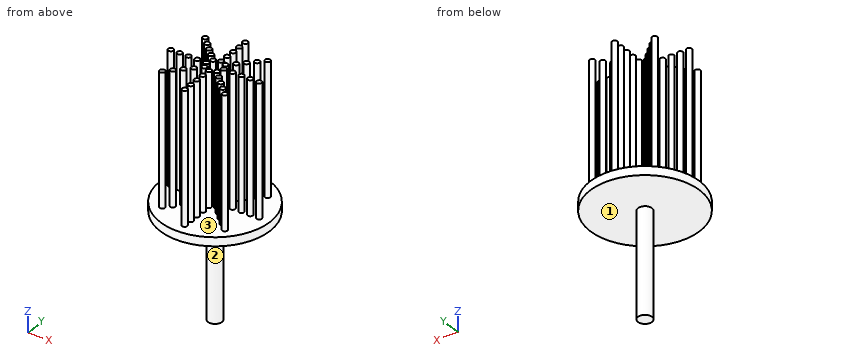
```python
from build123d import *

# Parameters (mm, degrees)
F0_R            = 62.5
F1_DEPTH        = 10
F2_R            = 3
F3_DEPTH        = 150
F3_COPIES_COUNT = 8
F4_R            = 8
F5_DEPTH        = 120


# Not quite as in the source:
# - a pattern or mirror of a feature is missing from the dataset's text; its kind, count and spacing are read off the source's solid


with BuildPart() as f1:
    # F0 (on Top) → F1 (new body)
    with BuildSketch(Plane.XY):
        Circle(F0_R)
    extrude(amount=F1_DEPTH)

    # F2 (on face) → F3 (join)
    with BuildSketch(Plane.XY.offset(10)):
        with Locations((10, 0)):
            Circle(F2_R)
        with Locations((20, 0)):
            Circle(F2_R)
        with Locations((30, 0)):
            Circle(F2_R)
        with Locations((40, 0)):
            Circle(F2_R)
        with Locations((50, 0)):
            Circle(F2_R)
    f3 = extrude(amount=F3_DEPTH)

    # F3_copies: F3 ×8 about axis
    f3_copies_axis = Axis((0, 0, 0), (0, 0, 1))
    for i in range(1, F3_COPIES_COUNT):
        add(f3.rotate(f3_copies_axis, i * 360 / F3_COPIES_COUNT))

    # F4 (on face) → F5 (join)
    with BuildSketch(Plane.XY):
        Circle(F4_R)
    extrude(amount=-F5_DEPTH)


solid = f1.part
```
Verification items for the finished model (mm, model axes). Face numbers are marked on the shaded views. Coordinates: 2 decimals unless noted, no trailing zeros. Order: outer loops, then holes, each group sorted by start corner. A loop starts at its lowest first (then second) coordinate and runs counter-clockwise, first axis right, second up. Notation, with made-up numbers: (87.5, 77.25) -> (126.5, 77.25) arc R21 cw to (126.5, 85.25) -> close; hole circle Ø3 at (-3, 19.25). An arc over 180 degrees is marked (long way). Answer as CSV lines item,"result". Start each with the question number.
1) Cross-section at C-C, the plane z = 104. Give the number of separate pieces and of enclosed holes in the cut face, then the cut area to 3 significant figures.
2) Release check for a two-part mould opening along Y. For the marked faces 1, 2 and 3 record: released by +Y, released by -Y, zero draft, split by the parting line, or undercut.
3) Gauge pin test, flat ends, axial feed: pin 1 Ø5 at (x, z) = (-6, -88) entering from +Y; pin 2 Ø6 at (x, z) = (-44.5, 62) entering from +Y; pin 3 Ø8 at (x, z) = (8.5, -71) entering from +Y. Record the tip position at first contact, or that the pin passes through.
4) Cross-section at A-A, the plane x = 50. Record the boundary of the cut face in (y, z), then the cut area to 3 significant figures.
5) Material ranges on L1, parallel to Y at x = 35, z = 46; L2, parallel to Y at x = 38, z = 44; L3, parallel to Z at x = -6.5, y = -6, recorded low to high. Write a range as [from, to].
Conclusion:
1,separate pieces,"40"
1,enclosed holes,"0"
1,area,"1,130 mm²"
2,face 1,"zero draft"
2,face 2,"split by the parting line"
2,face 3,"undercut"
3,pin 1,"stops at y = 7.19"
3,pin 2,"stops at y = 2.6"
3,pin 3,"stops at y = 6.61"
4,outline,"(-37.5, 0) -> (37.5, 0) -> (37.5, 10) -> (3, 10) -> (3, 160) -> (-3, 160) -> (-3, 10) -> (-37.5, 10) -> close"
4,area,"1,650 mm²"
5,L1,"y = [-38.33, -32.38], [32.38, 38.33]"
5,L2,"y = [-36.77, -33.94], [-2.24, 2.24], [33.94, 36.77]"
5,L3,"z = [0, 160]"
